Could you check a few things on this model? Use its own coordinates, in mm. A direction names the side the tool comes from. Round coordinates to 2 decimals unless told otherwise and drop trailing zeros. Loops run counter-clockwise (first coordinate to the right, second up) from the corner with the lowest first, then second, coordinate; pieces in that order, holes last. Notation, with made-up numbers: M -35,76.5 L -6,76.5 A24 ccw -6,89.5 Z; hole C -34,33.5 d10. An arc over 180 degrees is marked long. Answer in a Markdown table with one row per item.
```python
from build123d import *

# Parameters (mm, degrees)
SKETCH1_W                   = 50.8
SKETCH1_H                   = 12.7
BOSS_EXTRUDE1_DEPTH         = 25.4
F_1_4_28_TAPPED_HOLE1_D     = 5.4102
F_1_4_28_TAPPED_HOLE1_DEPTH = 29.972
F_1_4_28_TAPPED_HOLE1_TIP   = 1.625388061


with BuildPart() as part:
    # Sketch1 → Boss-Extrude1 (new body)
    with BuildSketch(Plane(origin=(0, 0, 0), x_dir=(1, 0, 0), z_dir=(0, 1, 0))):
        Rectangle(SKETCH1_W, SKETCH1_H)
    extrude(amount=BOSS_EXTRUDE1_DEPTH)

    # 1/4-28 Tapped Hole1
    with Locations(Plane(origin=(25.4, 0, 0), x_dir=(0, 0, -1), z_dir=(1, 0, 0))):
        with Locations((0, 6.215198177)):
            Hole(F_1_4_28_TAPPED_HOLE1_D / 2, depth=F_1_4_28_TAPPED_HOLE1_DEPTH)
            with Locations((0, 0, -(F_1_4_28_TAPPED_HOLE1_DEPTH + F_1_4_28_TAPPED_HOLE1_TIP / 2))):  # 118° drill point
                Cone(0, F_1_4_28_TAPPED_HOLE1_D / 2, F_1_4_28_TAPPED_HOLE1_TIP, mode=Mode.SUBTRACT)


solid = part.part
```
1) I need wall thicknesses on line 1 (Y direction, x = 3, z = 0); line 2 (Z direction, x = 19.5, y = 8.5). Which ranges of each line are inside material? Lowest first, please.
Computed:
| item | result |
|---|---|
| line 1 | y = 0 to 3.51, 8.92 to 25.4 |
| line 2 | z = -6.35 to -1.45, 1.45 to 6.35 |
2) If we mould it in two halves opening along Z, with no side actions, what happens to faces 3 (the face through (0, 13, -6.35)), 4 (the face through (-5.915, 5.757, 0.102)), 5 (the face through (-25.4, 13, 0))? For each: released by +Z, released by -Z, zero draft, split by the parting line, or undercut.
Computed:
| item | result |
|---|---|
| face 3 | released by -Z |
| face 4 | undercut |
| face 5 | zero draft |
3) I want a section at A-A, the plane x = 2.5. Please give me the cut outline in (y, z).
Computed:
| item | result |
|---|---|
| outline | M 0,-6.35 L 25.4,-6.35 L 25.4,6.35 L 0,6.35 Z; hole C 6.22,0 d5.41 |
4) Will this pin go through, and if not, where does the flat tip stop? P1, Ø4.5, axis at y = 6.22, z = 0, coming from the +X side.
Computed:
| item | result |
|---|---|
| P1 | stops at x = -4.84 |
5) Which directions (+Z, -Z, +X, -X, +Y, -Y) give clear straight access to the entire face, cutting with the end or side of a thin tool? Please do faces 1 (the face through (0, 0, 0)), 2 (the face through (10.2, 8.5, 1.45)).
Computed:
| item | result |
|---|---|
| face 1 | +Z, -Z, +X, -X, -Y |
| face 2 | +X |
